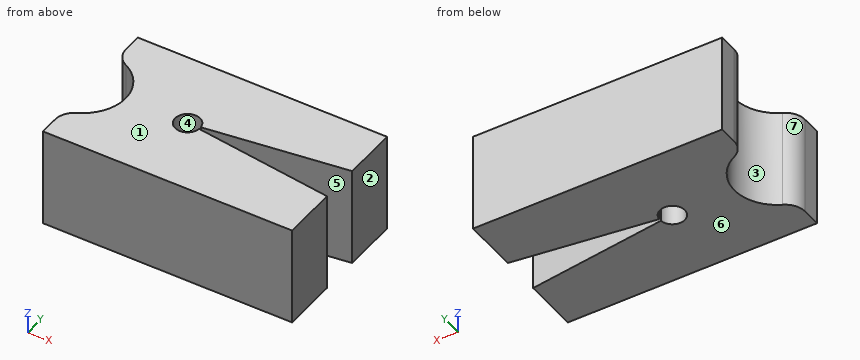
```python
from build123d import *

# Parameters (mm, degrees)
F0_W     = 63.5
F0_H     = 38.1
F1_DEPTH = 25.4
F4_DEPTH = 38.1
F5_R     = 10.795
F6_DEPTH = 38.1
F7_R     = 5.08


with BuildPart() as f1:
    # F0 (on Top) → F1 (new body)
    with BuildSketch(Plane.XY):
        Rectangle(F0_W, F0_H)
    extrude(amount=F1_DEPTH)

    # F3 (on face) → F4 (cut)
    with BuildSketch(Plane.XY.offset(25.4)):
        with BuildLine():
            Line((-3.8278593449, -0.3362854207), (-6.35, 0))
            Line((-6.35, 0), (-3.8278593449, 0.3362854207))
            ThreePointArc((-3.8278593449, 0.3362854207), (-10.16, 0), (-3.8278593449, -0.3362854207))
        make_face()
        with BuildLine():
            Line((-3.8278593449, 0.3362854207), (-6.35, 0))
            Line((-6.35, 0), (-3.8278593449, -0.3362854207))
            ThreePointArc((-3.8278593449, -0.3362854207), (-3.81446798, -0.1683796606), (-3.81, 0))
            ThreePointArc((-3.81, 0), (-3.81446798, 0.1683796606), (-3.8278593449, 0.3362854207))
        make_face()
        with BuildLine():
            Line((31.75, 5.08), (-3.8278593449, 0.3362854207))
            ThreePointArc((-3.8278593449, 0.3362854207), (-3.81446798, 0.1683796606), (-3.81, 0))
            ThreePointArc((-3.81, 0), (-3.81446798, -0.1683796606), (-3.8278593449, -0.3362854207))
            Line((-3.8278593449, -0.3362854207), (31.75, -5.08))
            Line((31.75, -5.08), (31.75, 5.08))
        make_face()
    extrude(amount=-F4_DEPTH, mode=Mode.SUBTRACT)

    # F5 (on face) → F6 (cut)
    with BuildSketch(Plane.XY.offset(25.4)):
        with Locations((-33.5856959183, 0)):
            Circle(F5_R)
    extrude(amount=-F6_DEPTH, mode=Mode.SUBTRACT)

    # F7
    f7_edges = [f1.edges().sort_by_distance(p)[0] for p in [
        (-31.75, 10.637774, 12.7),
        (-31.75, -10.637774, 12.7),
    ]]
    fillet(f7_edges, radius=F7_R)


solid = f1.part
```
Model file for the job. Use its own axes, mm. Face numbers are marked on the shaded views. A direction names the side the tool comes from. Coordinates: 2 decimals unless noted, no trailing zeros. Order: outer loops, then holes, each group sorted by start corner. A loop starts at its lowest first (then second) coordinate and runs counter-clockwise, first axis right, second up. Notation, with made-up numbers: (8, 89.25) -> (20, 89.25) arc R19 ccw to (20, 119.25) -> close; hole circle Ø1 at (3, -28). An arc over 180 degrees is marked (long way). Answer as a JSON object with one key per item and string values. Group by question number.
1) Which spindle directions (+Z, -Z, +X, -X, +Y, -Y) get a long thin tool onto all of the face, cutting with end or side? Do the marked faces 5, 6 and 7. Say none if no direction does.
2) Flat gauge pin, fed straight in: pin 1 (4 mm diameter, centred on y = -1.5, z = 14, fed in from -X). Where does the tip first touch, or does it go through?
3) Cut at A-A, the plane x = 8.5. Write the cut outline in (y, z).
4) Cut at C-C, the plane y = -2.5. Write the cut outline in (x, z), then the cut area to 3 significant figures.
5) Cut at D-D, the plane y = 7. Write the cut outline in (x, z).
6) Cut at B-B, the plane z = 13.25. Write the cut outline in (x, y) (3 decimals), then the cut area to 3 significant figures.
7) Pull direction X, two halves, no side cores. Call the marked faces 1, 2, 3 and 4: +X half, -X half, draft (parallel to the pull), parting line (faces both ways), or undercut.
8) Drill centre lines: L1, parallel to Y at x = 4, z = 13.25; L2, parallel to Y at x = -2.5, z = 15; L3, parallel to X at y = 0, z = 18. Where is each one in solid material? Low to high.
Check values:
{
 "1": {"face 5": "+Z, -Z, +X", "face 6": "-Z, +X, -X, +Y, -Y", "face 7": "+Z, -Z, -X"},
 "2": {"pin 1": "stops at x = -23.37"},
 "3": {"outline": "(-19.05, 0) -> (-1.98, 0) -> (-1.98, 25.4) -> (-19.05, 25.4) -> close; (1.98, 0) -> (19.05, 0) -> (19.05, 25.4) -> (1.98, 25.4) -> close"},
 "4": {"outline": "(-23.08, 0) -> (-8.94, 0) -> (-8.94, 25.4) -> (-23.08, 25.4) -> close; (-5.03, 0) -> (12.4, 0) -> (12.4, 25.4) -> (-5.03, 25.4) -> close", "area": "802 mm²"},
 "5": {"outline": "(-25.37, 0) -> (31.75, 0) -> (31.75, 25.4) -> (-25.37, 25.4) -> close"},
 "6": {"outline": "(-31.75, -19.05) -> (31.75, -19.05) -> (31.75, -5.08) -> (-3.828, -0.336) arc R3.175 cw (long way) to (-3.828, 0.336) -> (31.75, 5.08) -> (31.75, 19.05) -> (-31.75, 19.05) -> (-31.75, 14.289) arc R5.08 ccw to (-28.883, 9.717) arc R10.795 cw to (-28.883, -9.717) arc R5.08 ccw to (-31.75, -14.289) -> close", "area": "2,050 mm²"},
 "7": {"face 1": "draft", "face 2": "+X half", "face 3": "-X half", "face 4": "undercut"},
 "8": {"L1": "y = -19.05 to -1.38, 1.38 to 19.05", "L2": "y = -19.05 to -0.51, 0.51 to 19.05", "L3": "x = -22.79 to -10.16"}
}
